Input: dimensioned drawing with shaded views. Units: mm. Origin: part minimum x, y, z. Round coordinates to 2 decimals unless told otherwise and drop trailing zeros. Loops run counter-clockwise (first coordinate to the right, second up) from the corner with the lowest first, then second, coordinate; pieces in that order, holes last. Notation, with made-up numbers: M -28,32 L 21,32 A35 cw 21,65 Z; hole C 16.5,-20.5 d4. An arc over 180 degrees is marked long. Use one line per item in the form item = value. Start each with the question number.
Q1. Section query B-B, the plane y = 32. Output: boundary loops of the cut face in (x, z).
Q2. First-contact query: P1, Ø6, axis at y = 16.52, z = 46.1, coming from the +X side; P2, Ø16, axis at x = 66.5, z = 36, coming from the +Y side; P3, Ø9, axis at x = 98, y = 34.5, coming from the -Z side. Flat tips, straight axial feed; report the tip coordinate or a pass-through.
Q3. Section query A-A, the plane x = 110.5. Output: boundary loops of the cut face in (y, z), and give its area (3 significant figures).
Q4. Ray query, line 1 along X through (y, z) = (11.5, 29); line 2 along Z through (x, y) = (130, 9.5); line 3 along Y through (x, z) = (45, 31). Return the intervals inside material, ascending.
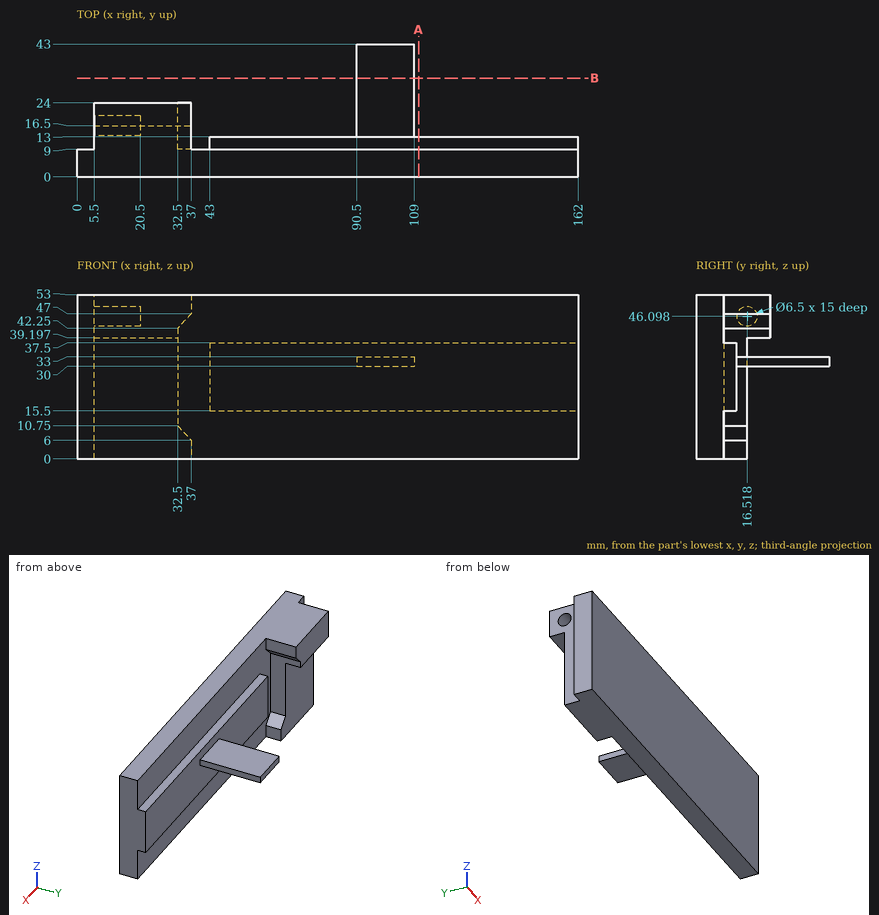
Results found:
q1.outline = M 90.5,30 L 109,30 L 109,33 L 90.5,33 Z
q2.P1 = 37
q2.P2 = 13
q2.P3 = 30
q3.outline = M 0,0 L 9,0 L 9,15.5 L 13,15.5 L 13,37.5 L 9,37.5 L 9,53 L 0,53 Z
q3.area = 565 mm²
q4.line_1 = 5.5 to 32.5, 43 to 162
q4.line_2 = 15.5 to 37.5
q4.line_3 = 0 to 13
